Input: part model. Units: mm. Frame: model coordinates. A direction names the side the tool comes from. Round coordinates to 2 decimals unless told otherwise and drop trailing zeros. Loops run counter-clockwise (first coordinate to the right, second up) from the corner with the lowest first, then second, coordinate; pieces in that order, holes last.
(1) Line query: line 1 (X direction, y = 2, z = -1.85); line 2 (X direction, y = -31, z = -0.4); line 3 (Y direction, x = -52.5, z = 0.55). Output: solid intervals per line, ascending.
(2) Draft query along Y for faces 1 (the face through (-45, -38.611, -1)), 2 (the face through (29.409, -36.764, -0.721)), 3 (the face through (-119.832, 0, -1)), 4 (the face through (5.62, -5.06, -0.72)). Return one class per face: released by +Y, released by -Y, zero draft, split by the parting line, or undercut.
(3) Access query for faces 5 (the face through (32.107, 0, -1)), 6 (the face through (-110.914, 2, -1)). Directions: +Z, -Z, +X, -X, +Y, -Y. A direction counts if a zero-diameter tool reaches every point of the face in a straight line with its end or side. Return the directions, or none.
(4) Cut plane B-B, the plane x = -34.5. Output: boundary loops of the cut face in (y, z).
(5) Cut plane A-A, the plane x = -67. Output: boundary loops of the cut face in (y, z), and give its area (3 significant figures).
(6) First-contact query: pin 1 Ø3 at (x, y) = (5.85, -6.8) entering from +Z. Flat tip, straight axial feed; report the tip coordinate or a pass-through.
(7) Cut plane C-C, the plane z = -0.2. Give the number of separate pieces and of enclosed holes in the cut face, and give its area (4 significant figures).
from build123d import *

# Parameters (mm, degrees)
ESQUISSE1_W        = 151.93976922
ESQUISSE1_H        = 78.51687395
ESQUISSE1_R        = 2
ESQUISSE1_R_2      = 4
ESQUISSE1_R_3      = 1.75
ESQUISSE1_R_4      = 3.75
ESQUISSE1_R_5      = 3.1
ESQUISSE1_W_2      = 86.5
ESQUISSE1_H_2      = 51.2
ESQUISSE1_W_3      = 5.937566171
ESQUISSE1_H_3      = 25.632907614
BOSS_EXTRU_1_DEPTH = 3


with BuildPart() as part:
    # Esquisse1 → Boss.-Extru.1 (new body)
    with BuildSketch(Plane.XY.offset(-2.2)):
        with Locations((-43.862390942, 0.647054174)):
            Rectangle(ESQUISSE1_W, ESQUISSE1_H)
        with Locations((-109.194417438, 24.821428571)):
            Circle(ESQUISSE1_R, mode=Mode.SUBTRACT)
        with Locations((-109.194417438, -21.178571429)):
            Circle(ESQUISSE1_R, mode=Mode.SUBTRACT)
        with Locations((-1.194417438, -21.178571429)):
            Circle(ESQUISSE1_R, mode=Mode.SUBTRACT)
        with Locations((-1.194417438, 24.821428571)):
            Circle(ESQUISSE1_R, mode=Mode.SUBTRACT)
        with Locations((-116.210955208, 36.284170806)):
            Circle(ESQUISSE1_R, mode=Mode.SUBTRACT)
        with Locations((-116.210955208, -34.990062458)):
            Circle(ESQUISSE1_R, mode=Mode.SUBTRACT)
        with Locations((28.486173324, 36.284170806)):
            Circle(ESQUISSE1_R, mode=Mode.SUBTRACT)
        with Locations((28.486173324, -34.990062458)):
            Circle(ESQUISSE1_R, mode=Mode.SUBTRACT)
        with Locations((14.345224597, 6.749852674)):
            Circle(ESQUISSE1_R_2, mode=Mode.SUBTRACT)
        with Locations((5.845224597, 16.204342535)):
            Circle(ESQUISSE1_R_3, mode=Mode.SUBTRACT)
        with Locations((22.845224597, 16.204342535)):
            Circle(ESQUISSE1_R_3, mode=Mode.SUBTRACT)
        with Locations((22.845224597, -6.795657465)):
            Circle(ESQUISSE1_R_3, mode=Mode.SUBTRACT)
        with Locations((5.845224597, -6.795657465)):
            Circle(ESQUISSE1_R_3, mode=Mode.SUBTRACT)
        with Locations((14.176552179, -18.611382801)):
            Circle(ESQUISSE1_R_4, mode=Mode.SUBTRACT)
        with Locations((-79.237508709, -31.316718293)):
            Circle(ESQUISSE1_R_5, mode=Mode.SUBTRACT)
        with Locations((-35.905557573, -31.316718293)):
            Circle(ESQUISSE1_R_5, mode=Mode.SUBTRACT)
        with Locations((-52.444417438, 1.821428571)):
            Rectangle(ESQUISSE1_W_2, ESQUISSE1_H_2, mode=Mode.SUBTRACT)
        with Locations((-107.94493025, 1.811094224)):
            Rectangle(ESQUISSE1_W_3, ESQUISSE1_H_3, mode=Mode.SUBTRACT)
    extrude(amount=BOSS_EXTRU_1_DEPTH)


solid = part.part
Reported:
1. line 1: x = -119.83 to -110.91, -104.98 to -95.69, -9.19 to 32.11
1. line 2: x = -119.83 to -82.32, -76.15 to -38.99, -32.82 to 32.11
1. line 3: y = -38.61 to -23.78, 27.42 to 39.91
2. face 1: released by -Y
2. face 2: undercut
2. face 3: zero draft
2. face 4: undercut
3. face 5: +Z, -Z, +X, +Y, -Y
3. face 6: +Z, -Z
4. outline: (-38.61, -2.2) - (-34.08, -2.2) - (-34.08, 0.8) - (-38.61, 0.8) - close; (-28.55, -2.2) - (-23.78, -2.2) - (-23.78, 0.8) - (-28.55, 0.8) - close; (27.42, -2.2) - (39.91, -2.2) - (39.91, 0.8) - (27.42, 0.8) - close
5. outline: (-38.61, -2.2) - (-23.78, -2.2) - (-23.78, 0.8) - (-38.61, 0.8) - close; (27.42, -2.2) - (39.91, -2.2) - (39.91, 0.8) - (27.42, 0.8) - close
5. area: 82.0 mm2
6. pin 1: passes through
7. separate pieces: 1
7. enclosed holes: 18
7. area: 7,055 mm2
